For this review, take the finished solid that the model builds, in its own axes (mm). Round coordinates to 2 decimals unless told otherwise and drop trailing zeros. Loops run counter-clockwise (first coordinate to the right, second up) from the corner with the lowest first, then second, coordinate; pieces in that order, holes last. Notation, with made-up numbers: (43, 72.25) -> (96, 72.25) arc R24 ccw to (96, 88.25) -> close; hole circle Ø3 at (63.5, -0.75). An arc over 180 degrees is marked (long way). Write each question's results on one line, items separated by ' | '.
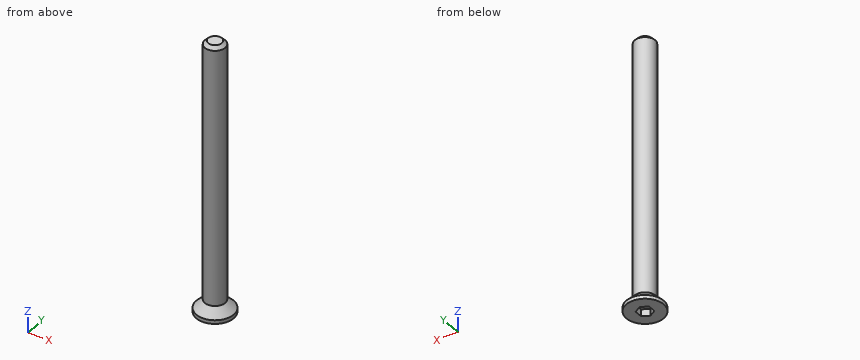
Autodesk Inventor part; units mm, degrees
ref_plane "YZ Plane" through (0, 0, 0) normal (1, 0, 0) x (0, 1, 0)
ref_plane "XZ Plane" through (0, 0, 0) normal (0, 1, 0) x (-1, 0, 0)
ref_plane "XY Plane" through (0, 0, 0) normal (0, 0, 1) x (1, 0, 0)
sketch "Эскиз1" plane through (0, 0, 0) normal (0, 0, 1) x (1, 0, 0)
  circle A0 centre (0, 0) radius 1.5
  circle A1 centre (0, 0) radius 2.75
  line L0 (0, 1.1547) -> (1, 0.5774)
  line L1 (1, 0.5774) -> (1, -0.5774)
  line L2 (1, -0.5774) -> (0, -1.1547)
  line L3 (0, -1.1547) -> (-1, -0.5774)
  line L4 (-1, -0.5774) -> (-1, 0.5774)
  line L5 (-1, 0.5774) -> (0, 1.1547)
  dimension "d0" = 3
  dimension "d1" = 5.5
  dimension "d2" = 2
extrude "Выдавливание1" add sketch "Эскиз1" along normal blind 40 contours A0 | L0 L1 L2 L3 L4 L5
extrude "Выдавливание2" add sketch "Эскиз1" along normal blind 1.8 contours A1
chamfer "Фаска1" distance 1.25 angle 45 1 edges at (-2.75, 0, 1.8)
extrude "Выдавливание3" cut sketch "Эскиз1" along normal blind 1 contours L0 L1 L2 L3 L4 L5
chamfer "Фаска2" distance 0.5 angle 45 1 edges at (-1.5, 0, 40)
properties part number "M3X40"
1. Consider section B-B (z = 24). State the section outline as (x, y) points.
Values found:
outline: circle Ø3 at (0, 0)
2. For pin 1 (1 mm diameter, centred on y = 0, z = 32.5, fed in from +X); pin 2 (3 mm diameter, centred on x = 2, z = 13.5, fed in from -Y); pin 3 (1 mm diameter, centred on x = -1, y = -0.5, fed in from -Z), all flat-tipped, find the tip position at first contact; note any pin that passes through.
Values found:
pin 1: stops at x = 1.5 | pin 2: stops at y = -1.41 | pin 3: stops at z = 0
3. To check wall thickness, follow probe 1 along X at (y, z) = (0.1, 7.5); probe 2 along Z at (x, y) = (-1.1, -1.85); probe 3 along Z at (x, y) = (1.7, -0.6). State the ranges of each line that lie inside material, in increasing order.
Values found:
probe 1: x = -1.5 to 1.5 | probe 2: z = 0 to 1.15 | probe 3: z = 0 to 1.5
